Could you check a few things on this model? Use its own coordinates, in mm. Face numbers are marked on the shaded views. A direction names the side the tool comes from. Give positions to 0.01 mm unless a question says otherwise; leave off trailing zeros. Write each loop counter-clockwise with the first axis right and the second up, starting at its lowest first coordinate (ties: lowest second). Pieces come first, ordered by that corner, then holes. Notation, with made-up numbers: (-15, 10) - (27, 10) arc R6 cw to (27, 15) - close; hole circle Ø11 at (15.25, -26.5). An arc over 180 degrees is marked (long way). Use one line per item in the form item = value.
```python
from build123d import *

# Parameters (mm, degrees)
SKETCH1_W           = 55.372
SKETCH1_H           = 57.15
BOSS_EXTRUDE1_DEPTH = 34.29
SHELL1_T            = -3.175
CUT_EXTRUDE1_DEPTH  = 39.116


with BuildPart() as part:
    # Sketch1 → Boss-Extrude1 (new body)
    with BuildSketch(Plane.XY):
        with Locations((6.35, 5.207)):
            Rectangle(SKETCH1_W, SKETCH1_H)
    extrude(amount=BOSS_EXTRUDE1_DEPTH)

    # Shell1
    shell1_openings = [part.faces().sort_by_distance(p)[0] for p in [
        (6.35, 5.207, 34.29),
        (6.35, -23.368, 17.145),
    ]]
    offset(amount=SHELL1_T, openings=shell1_openings, kind=Kind.INTERSECTION)

    # Sketch2 → Cut-Extrude1 (cut)
    with BuildSketch(Plane.XZ.offset(-30.607)):
        Polygon((-18.161, 15.875), (10.564637788, 15.875), (30.861, 15.875), (30.861, 34.29), (-18.161, 34.29), align=None)
    extrude(amount=-CUT_EXTRUDE1_DEPTH, mode=Mode.SUBTRACT)


solid = part.part
```
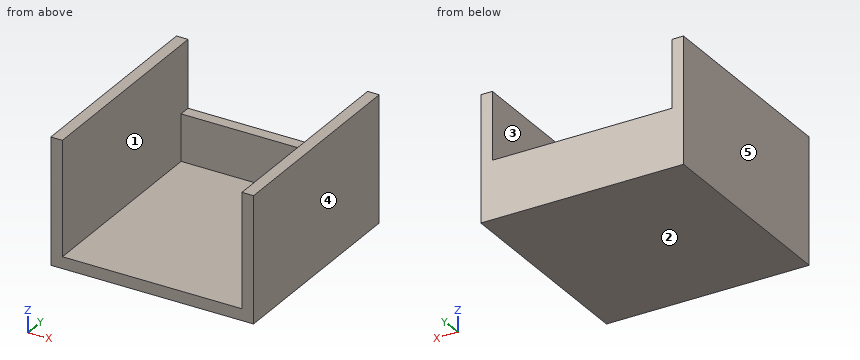
1. Imagine slicing it at D-D, the plane z = 5.5. List the corners of the cut face in (x, y) for me, and give its area (3 significant figures).
Response values:
outline = (-21.34, -23.37) - (-18.16, -23.37) - (-18.16, 30.61) - (30.86, 30.61) - (30.86, -23.37) - (34.04, -23.37) - (34.04, 33.78) - (-21.34, 33.78) - close
area = 519 mm²
2. Which directions (+Z, -Z, +X, -X, +Y, -Y) give clear straight access to the entire face, cutting with the end or side of a thin tool? Please do the marked faces 1 and 2.
Response values:
face_1 = +Z, -Y
face_2 = -Z, +X, -X, +Y, -Y
3. Imagine slicing it at A-A, the plane z = 27.5. List the corners of the cut face in (x, y) for me.
Response values:
outline = (-21.34, -23.37) - (-18.16, -23.37) - (-18.16, 33.78) - (-21.34, 33.78) - close; (30.86, -23.37) - (34.04, -23.37) - (34.04, 33.78) - (30.86, 33.78) - close
4. If we mould it in two halves opening along X, with no side actions, what happens to the marked faces 3, 4 and 5? For each: pulls with the +X half, pulls with the -X half, needs draft (parallel to the pull), parting line crosses it, or undercut.
Response values:
face_3 = undercut
face_4 = pulls with the +X half
face_5 = pulls with the -X half
5. For pin 1 (4 mm diameter, centred on x = 3, z = 10.5, fed in from -Y); pin 2 (24.5 mm diameter, centred on x = 10, y = 15.5, fed in from +Z) (3 decimals); pin 3 (3.5 mm diameter, centred on x = -0.5, y = 33, fed in from +Z) (3 decimals), each with a flat end and sliding along its axis, tell me the tip position at first contact or that it passes through.
Response values:
pin_1 = 30.61
pin_2 = 3.175
pin_3 = 15.875
6. If I drill on line 1 (X direction, y = -17, z = 29); line 2 (Z direction, x = -13, y = -14.5) (3 decimals); line 3 (Y direction, x = -4, z = 12), over which ranges is the centre line in solid material (lowest first)? Write a range as from..to.
Response values:
line_1 = -21.34..-18.16, 30.86..34.04
line_2 = 0..3.175
line_3 = 30.61..33.78
7. Imagine slicing it at B-B, the plane y = 9. List the corners of the cut face in (x, z) for me (3 decimals), and give its area (3 significant figures).
Response values:
outline = (-21.336, 0) - (34.036, 0) - (34.036, 34.29) - (30.861, 34.29) - (30.861, 3.175) - (-18.161, 3.175) - (-18.161, 34.29) - (-21.336, 34.29) - close
area = 373 mm²
8. Imagine slicing it at C-C, the plane x = 6.5. List the corners of the cut face in (y, z) for me (3 decimals).
Response values:
outline = (-23.368, 0) - (33.782, 0) - (33.782, 15.875) - (30.607, 15.875) - (30.607, 3.175) - (-23.368, 3.175) - close
